Verification items for the finished model (mm, model axes). A direction names the side the tool comes from. Give positions to 0.01 mm unless a question says otherwise; leave off trailing zeros. Write each loop counter-clockwise with the first axis right and the second up, starting at its lowest first coordinate (ties: lowest second). Pieces come first, ordered by that corner, then holes. Notation, with made-up numbers: (69, 8) - (90, 8) arc R24 ccw to (90, 26) - close; hole circle Ø3 at (-16, 58.5). An arc over 180 degrees is marked (long way). Put each result on its own line as item: value.
from build123d import *

# Parameters (mm, degrees)
SKETCH_1_R          = 1.65
EXTRUDE_1_DEPTH     = 4
EXTRUDE_START       = 1.5
SKETCH_1_3_R        = 1.65
SKETCH_1_3_W        = 91.5
SKETCH_1_3_H        = 77.5
SKETCH_1_3_W_2      = 85.9
SKETCH_1_3_H_2      = 64.9
SKETCH_1_3_W_3      = 17.5
SKETCH_1_3_H_3      = 2.5
EXTRUDE_2_DEPTH     = 1.5
FILLET_1_R          = 2
FILLET_2_R          = 1
CUT_EXTRUDE_START   = -4
CUT_EXTRUDE_1_DEPTH = 4
SKETCH_5_W          = 2.5
SKETCH_5_H          = 4.652730878
SKETCH_5_W_2        = 1
CUT_EXTRUDE_2_DEPTH = 1


with BuildPart() as part:
    # 草图1 → 凸台-拉伸1 (new body)
    with BuildSketch(Plane.XY):
        with BuildLine():
            Line((48.768130557, 44.382842821), (-48.768130557, 44.382842821))
            ThreePointArc((-48.768130557, 44.382842821), (-50.8894509, 43.504163165), (-51.768130557, 41.382842821))
            Line((-51.768130557, 41.382842821), (-51.768130557, -41.882842821))
            ThreePointArc((-51.768130557, -41.882842821), (-50.8894509, -44.004163165), (-48.768130557, -44.882842821))
            Line((-48.768130557, -44.882842821), (48.768130557, -44.882842821))
            ThreePointArc((48.768130557, -44.882842821), (50.8894509, -44.004163165), (51.768130557, -41.882842821))
            Line((51.768130557, -41.882842821), (51.768130557, 41.382842821))
            ThreePointArc((51.768130557, 41.382842821), (50.8894509, 43.504163165), (48.768130557, 44.382842821))
        make_face()
        with Locations((-48.268130557, -40.882842821)):
            Circle(SKETCH_1_R, mode=Mode.SUBTRACT)
        Polygon((-45.75, -38.75), (-45.75, 38.75), (45.75, 38.75), (45.75, -38.75), (8.75, -38.75), (8.75, -41.25), (-8.75, -41.25), (-8.75, -38.75), align=None, mode=Mode.SUBTRACT)
        with Locations((48.268130557, -40.882842821)):
            Circle(SKETCH_1_R, mode=Mode.SUBTRACT)
        with Locations((-48.268130557, 40.882842821)):
            Circle(SKETCH_1_R, mode=Mode.SUBTRACT)
        with Locations((48.268130557, 40.882842821)):
            Circle(SKETCH_1_R, mode=Mode.SUBTRACT)
    extrude(amount=-EXTRUDE_1_DEPTH)

    # 草图1<3> → 凸台-拉伸2 (add)
    # profile 1 of 7: a face of its own
    with BuildSketch(Plane.XY.offset(EXTRUDE_START)):
        with BuildLine():
            Line((-48.768130557, 44.382842821), (48.768130557, 44.382842821))
            ThreePointArc((48.768130557, 44.382842821), (50.8894509, 43.504163165), (51.768130557, 41.382842821))
            Line((51.768130557, 41.382842821), (51.768130557, -41.882842821))
            ThreePointArc((51.768130557, -41.882842821), (50.8894509, -44.004163165), (48.768130557, -44.882842821))
            Line((48.768130557, -44.882842821), (-48.768130557, -44.882842821))
            ThreePointArc((-48.768130557, -44.882842821), (-50.8894509, -44.004163165), (-51.768130557, -41.882842821))
            Line((-51.768130557, -41.882842821), (-51.768130557, 41.382842821))
            ThreePointArc((-51.768130557, 41.382842821), (-50.8894509, 43.504163165), (-48.768130557, 44.382842821))
        make_face()
        with Locations((48.268130557, 40.882842821)):
            Circle(SKETCH_1_3_R, mode=Mode.SUBTRACT)
        with Locations((-48.268130557, 40.882842821)):
            Circle(SKETCH_1_3_R, mode=Mode.SUBTRACT)
        with Locations((-48.268130557, -40.882842821)):
            Circle(SKETCH_1_3_R, mode=Mode.SUBTRACT)
        with Locations((48.268130557, -40.882842821)):
            Circle(SKETCH_1_3_R, mode=Mode.SUBTRACT)
        Rectangle(SKETCH_1_3_W, SKETCH_1_3_H, mode=Mode.SUBTRACT)
    # profile 2 of 7: a face of its own
    with BuildSketch(Plane.XY.offset(EXTRUDE_START)):
        with Locations((-48.268130557, -40.882842821)):
            Circle(SKETCH_1_3_R)
    # profile 3 of 7: a face of its own
    with BuildSketch(Plane.XY.offset(EXTRUDE_START)):
        with Locations((48.268130557, -40.882842821)):
            Circle(SKETCH_1_3_R)
    # profile 4 of 7: a face of its own
    with BuildSketch(Plane.XY.offset(EXTRUDE_START)):
        with Locations((48.268130557, 40.882842821)):
            Circle(SKETCH_1_3_R)
    # profile 5 of 7: a face of its own
    with BuildSketch(Plane.XY.offset(EXTRUDE_START)):
        with Locations((-48.268130557, 40.882842821)):
            Circle(SKETCH_1_3_R)
    # profile 6 of 7: a face of its own
    with BuildSketch(Plane.XY.offset(EXTRUDE_START)):
        Rectangle(SKETCH_1_3_W, SKETCH_1_3_H)
        with Locations((0, 3.3)):
            Rectangle(SKETCH_1_3_W_2, SKETCH_1_3_H_2, mode=Mode.SUBTRACT)
    # profile 7 of 7: a face of its own
    with BuildSketch(Plane.XY.offset(EXTRUDE_START)):
        with Locations((0, -40)):
            Rectangle(SKETCH_1_3_W_3, SKETCH_1_3_H_3)
    extrude(amount=-EXTRUDE_2_DEPTH)

    # 圆角1
    fillet_1_edges = [part.edges().sort_by_distance(p)[0] for p in [
        (0, 44.382842821, 1.5),
        (50.8894509, -44.004163165, 1.5),
        (51.768130557, -0.25, 1.5),
        (-50.8894509, 43.504163165, 1.5),
        (-51.768130557, -0.25, 1.5),
        (-50.8894509, -44.004163165, 1.5),
        (0, -44.882842821, 1.5),
        (50.8894509, 43.504163165, 1.5),
    ]]
    fillet(fillet_1_edges, radius=FILLET_1_R)

    # 圆角2
    fillet_2_edges = [part.edges().sort_by_distance(p)[0] for p in [
        (0, -41.25, -4),
        (-27.25, -38.75, -4),
        (-45.75, 0, -4),
        (0, 38.75, -4),
        (45.75, 0, -4),
        (27.25, -38.75, -4),
    ]]
    fillet(fillet_2_edges, radius=FILLET_2_R)

    # 草图2 → 切除-拉伸1 (cut)
    with BuildSketch(Plane(origin=(0, 0, -4), x_dir=(-1, 0, 0), z_dir=(0, 0, -1)).offset(CUT_EXTRUDE_START)):
        with BuildLine():
            Line((-46.015064843, 36.8), (-45.484935157, 36.8))
            ThreePointArc((-45.484935157, 36.8), (-41.25, 35), (-45.484935157, 33.2))
            Line((-45.484935157, 33.2), (-46.015064843, 33.2))
            ThreePointArc((-46.015064843, 33.2), (-50.25, 35), (-46.015064843, 36.8))
        make_face()
        with BuildLine():
            Line((46.015064843, 33.2), (45.484935157, 33.2))
            ThreePointArc((45.484935157, 33.2), (41.25, 35), (45.484935157, 36.8))
            Line((45.484935157, 36.8), (46.015064843, 36.8))
            ThreePointArc((46.015064843, 36.8), (50.25, 35), (46.015064843, 33.2))
        make_face()
        with BuildLine():
            Line((46.015064843, -36.8), (45.484935157, -36.8))
            ThreePointArc((45.484935157, -36.8), (41.25, -35), (45.484935157, -33.2))
            Line((45.484935157, -33.2), (46.015064843, -33.2))
            ThreePointArc((46.015064843, -33.2), (50.25, -35), (46.015064843, -36.8))
        make_face()
        with BuildLine():
            Line((-46.015064843, -33.2), (-45.484935157, -33.2))
            ThreePointArc((-45.484935157, -33.2), (-41.25, -35), (-45.484935157, -36.8))
            Line((-45.484935157, -36.8), (-46.015064843, -36.8))
            ThreePointArc((-46.015064843, -36.8), (-50.25, -35), (-46.015064843, -33.2))
        make_face()
    extrude(amount=CUT_EXTRUDE_1_DEPTH, mode=Mode.SUBTRACT)

    # 扫描1: sweep along a path in 草图3
    with BuildLine(Plane(origin=(0, 0, 0), x_dir=(-1, 0, 0), z_dir=(0, 0, -1))) as sweep_1_path:
        Line((41.45, 34.25), (41.45, -27.65))
        Line((41.45, -27.65), (-41.45, -27.65))
        Line((-41.45, -27.65), (-41.45, 34.25))
        Line((-41.45, 34.25), (41.45, 34.25))
    # 草图4 → 扫描1 (sweep)
    with BuildSketch(Plane(origin=(0, 0, 0), x_dir=(1, 0, 0), z_dir=(0, 1, 0))):
        with BuildLine():
            Line((41.45, 0), (42.95, 0))
            Line((42.95, 0), (42.95, -1.5))
            ThreePointArc((42.95, -1.5), (41.889339828, -1.060660172), (41.45, 0))
        make_face()
    sweep(path=sweep_1_path.line, transition=Transition.RIGHT)

    # 草图5 → 切除-拉伸2 (cut)
    with BuildSketch(Plane(origin=(0, 0, -4), x_dir=(-1, 0, 0), z_dir=(0, 0, -1))):
        with Locations((48, 7.013523993)):
            Rectangle(SKETCH_5_W, SKETCH_5_H)
        with Locations((46.25, 7.013523993)):
            Rectangle(SKETCH_5_W_2, SKETCH_5_H)
    extrude(amount=-CUT_EXTRUDE_2_DEPTH, mode=Mode.SUBTRACT)


solid = part.part
Q1. Section check C-C, the plane y = -35. Record the cut outline in (x, z).
Answers follow:
outline: (-51.77, -4) - (-50.25, -4) - (-50.25, 0) - (50.25, 0) - (50.25, -4) - (51.77, -4) - (51.77, -0.5) arc R2 ccw to (49.77, 1.5) - (-49.77, 1.5) arc R2 ccw to (-51.77, -0.5) - close
Q2. Section check B-B, the plane x = -23. Record the cut outline in (y, z).
Answers follow:
outline: (-44.88, -4) - (-39.75, -4) arc R1 ccw to (-38.75, -3) - (-38.75, 0) - (-27.65, 0) arc R1.5 ccw to (-29.15, 1.5) - (-42.88, 1.5) arc R2 ccw to (-44.88, -0.5) - close; (34.25, 0) - (38.75, 0) - (38.75, -3) arc R1 ccw to (39.75, -4) - (44.38, -4) - (44.38, -0.5) arc R2 ccw to (42.38, 1.5) - (35.75, 1.5) arc R1.5 ccw to start
Q3. Section check D-D, the plane z = -1.35. Give the number of separate pieces and of enclosed holes in the cut face, plus the area to 3 significant figures.
Answers follow:
separate pieces: 1
enclosed holes: 5
area: 1,990 mm2
Q4. Set-up check for faces 4 (the face through (51.768, 0, -2)), 5 (the face through (-49.58, 39.88, -1.97)): record each of +Z, -Z, +X, -X, +Y, -Y from which the full face is reachable in a straight line by a thin tool's end or side.
Answers follow:
face 4: +Z, -Z, +X, +Y, -Y
face 5: -Z
Q5. Release check for a two-part mould opening along Y. For faces 1 (the face through (1, -44.883, -2)), 2 (the face through (-51.768, -1, -2)), 3 (the face through (50.25, -35.08, -1.97)) record: released by +Y, released by -Y, zero draft, split by the parting line, or undercut.
Answers follow:
face 1: released by -Y
face 2: zero draft
face 3: undercut
Q6. Section check A-A, the plane y = 17. Record the cut outline in (x, z).
Answers follow:
outline: (-51.77, -4) - (-46.75, -4) arc R1 ccw to (-45.75, -3) - (-45.75, 0) - (-41.45, 0) arc R1.5 ccw to (-42.95, 1.5) - (-49.77, 1.5) arc R2 ccw to (-51.77, -0.5) - close; (41.45, 0) - (45.75, 0) - (45.75, -3) arc R1 ccw to (46.75, -4) - (51.77, -4) - (51.77, -0.5) arc R2 ccw to (49.77, 1.5) - (42.95, 1.5) arc R1.5 ccw to start
Q7. Go/stop test with a flat-tipped pin: pin 1 Ø3 at (x, y) = (47.75, -35) entering from -Z. Record where the tip stops, or that it passes through.
Answers follow:
pin 1: stops at z = 0
Q8. Scan lines: line 1 along X through (y, z) = (4.5, -2.1); line 2 along X through (y, z) = (-40, -2.2); line 3 along Y through (x, z) = (31.5, -2.75). Record each from-to range of solid material in increasing order.
Answers follow:
line 1: x = -51.77 to -45.75, 45.75 to 51.77
line 2: x = -51.77 to -49.66, -46.87 to -8.75, 8.75 to 46.87, 49.66 to 51.77
line 3: y = -44.88 to -38.75, 38.75 to 44.38
